Input: part model. Units: mm. Frame: model coordinates. A direction names the side the tool comes from. Give positions to 0.01 mm unless a question says otherwise; leave off trailing zeros. Loops run counter-clockwise (first coordinate to the right, second up) from the corner with the lowest first, then second, coordinate; pieces in that order, holes last. Notation, with made-up numbers: M 86.25,87.25 L 93.25,87.25 A27 cw 93.25,116.25 Z; hole C 13.5,58.5 d10. An arc over 180 degrees is marked long. Answer as a JSON object with one key per item and string values. Group by question number.
```python
from build123d import *
from build123d.topology import SkipClean

# Parameters (mm, degrees)
SKETCH1_R               = 16.65
BOSS_EXTRUDE1_DEPTH     = 2.5
SKETCH2_R               = 15.15
BOSS_EXTRUDE2_DEPTH     = 1.3
SKETCH3_R               = 16.65
BOSS_EXTRUDE3_DEPTH     = 27
CUT_EXTRUDE1_DEPTH      = 27
CUT_EXTRUDE1_DEPTH_BACK = 27
CUT_EXTRUDE2_DEPTH      = 26
CUT_EXTRUDE3_DEPTH      = 12.5
BOSS_EXTRUDE4_START     = -7
SKETCH8_R               = 4
BOSS_EXTRUDE4_DEPTH     = 10.5
FILLET1_R               = 3
SKETCH9_R               = 4
CUT_EXTRUDE4_DEPTH      = 33.5
CUT_EXTRUDE5_DEPTH      = 2
SKETCH11_R              = 15.35
CUT_EXTRUDE6_DEPTH      = 4


with BuildPart() as part:
    # Sketch1 → Boss-Extrude1 (new body)
    with BuildSketch(Plane(origin=(0, 0, 0), x_dir=(1, 0, 0), z_dir=(0, 1, 0))):
        with Locations(Location((0, 0, 0), (0, 0, 270))):
            Circle(SKETCH1_R)
    extrude(amount=BOSS_EXTRUDE1_DEPTH)

    # Sketch2 → Boss-Extrude2 (add)
    with BuildSketch(Plane(origin=(0, 2.5, 0), x_dir=(1, 0, 0), z_dir=(0, 1, 0))):
        with Locations(Location((0, 0, 0), (0, 0, 270))):
            Circle(SKETCH2_R)
    extrude(amount=BOSS_EXTRUDE2_DEPTH)

    # Sketch3 → Boss-Extrude3 (add)
    with BuildSketch(Plane(origin=(0, 3.8, 0), x_dir=(1, 0, 0), z_dir=(0, 1, 0))):
        with Locations(Location((0, 0, 0), (0, 0, 270))):
            Circle(SKETCH3_R)
    extrude(amount=BOSS_EXTRUDE3_DEPTH)

    # Sketch4 → Cut-Extrude1 (cut, two sides: drawn at the far end of the back side and taken through both)
    with BuildSketch(Plane.XY.offset(-CUT_EXTRUDE1_DEPTH_BACK)):
        with BuildLine():
            Line((-12.15, 30.8), (-10.299201712, 28.949201712))
            ThreePointArc((-10.299201712, 28.949201712), (-9.001508317, 28.082110707), (-7.470774587, 27.777628837))
            Line((-7.470774587, 27.777628837), (7.470774587, 27.777628837))
            ThreePointArc((7.470774587, 27.777628837), (9.001508317, 28.082110707), (10.299201712, 28.949201712))
            Line((10.299201712, 28.949201712), (12.15, 30.8))
            Line((12.15, 30.8), (-12.15, 30.8))
        make_face()
    extrude(amount=CUT_EXTRUDE1_DEPTH + CUT_EXTRUDE1_DEPTH_BACK, mode=Mode.SUBTRACT)

    # Sketch6 → Cut-Extrude2 (cut)
    with BuildSketch(Plane(origin=(0, 30.8, 0), x_dir=(1, 0, 0), z_dir=(0, 1, 0))):
        with BuildLine():
            Line((-12.249897959, 9.25), (12.249897959, 9.25))
            ThreePointArc((12.249897959, 9.25), (15.35, 0), (12.249897959, -9.25))
            Line((12.249897959, -9.25), (-12.249897959, -9.25))
            ThreePointArc((-12.249897959, -9.25), (-15.35, 0), (-12.249897959, 9.25))
        make_face()
    extrude(amount=-CUT_EXTRUDE2_DEPTH, mode=Mode.SUBTRACT)

    # Sketch7 → Cut-Extrude3 (cut)
    with BuildSketch(Plane.XY.offset(24.5)):
        with BuildLine():
            Line((-9.3, 6.2), (9.3, 6.2))
            ThreePointArc((9.3, 6.2), (10.714213562, 6.785786438), (11.3, 8.2))
            Line((11.3, 8.2), (11.3, 19.5))
            ThreePointArc((11.3, 19.5), (10.714213562, 20.914213562), (9.3, 21.5))
            Line((9.3, 21.5), (-9.3, 21.5))
            ThreePointArc((-9.3, 21.5), (-10.714213562, 20.914213562), (-11.3, 19.5))
            Line((-11.3, 19.5), (-11.3, 8.2))
            ThreePointArc((-11.3, 8.2), (-10.714213562, 6.785786438), (-9.3, 6.2))
        make_face()
    cut_extrude3 = extrude(amount=-CUT_EXTRUDE3_DEPTH, mode=Mode.SUBTRACT)

    # Mirror1: Cut-Extrude3 across plane
    add(cut_extrude3.mirror(Plane.XY), mode=Mode.SUBTRACT)

    # Sketch8 → Boss-Extrude4 (add)
    with BuildSketch(Plane(origin=(0, 0, -12), x_dir=(-1, 0, 0), z_dir=(0, 0, -1)).offset(BOSS_EXTRUDE4_START)):
        with BuildLine():
            Line((-2.837252192, 21.5), (2.837252192, 21.5))
            ThreePointArc((2.837252192, 21.5), (0, 10), (-2.837252192, 21.5))
        make_face()
        with Locations((0, 16.1)):
            Circle(SKETCH8_R, mode=Mode.SUBTRACT)
    boss_extrude4 = extrude(amount=BOSS_EXTRUDE4_DEPTH)

    # Mirror2: Boss-Extrude4 across plane
    add(boss_extrude4.mirror(Plane.XY))

    # Fillet1
    fillet1_edges = [part.edges().sort_by_distance(p)[0] for p in [
        (15.35, 4.8, 0),
        (0, 4.8, 9.25),
        (-15.35, 4.8, 0),
        (0, 4.8, -9.25),
    ]]
    fillet(fillet1_edges, radius=FILLET1_R)

    # Sketch9 → Cut-Extrude4 (cut)
    with BuildSketch(Plane(origin=(0, 0, -12), x_dir=(-1, 0, 0), z_dir=(0, 0, -1))):
        with Locations((0, 16.1)):
            Circle(SKETCH9_R)
    extrude(amount=-CUT_EXTRUDE4_DEPTH, mode=Mode.SUBTRACT)

    # Sketch10 → Cut-Extrude5 (cut)
    with SkipClean():  # the faces are left unmerged after this step: merging them gives an invalid solid
        with BuildSketch(Plane(origin=(0, 0, -12), x_dir=(-1, 0, 0), z_dir=(0, 0, -1))):
            with BuildLine():
                Line((0.611782833, 6.2), (0.611782833, 10.03075608))
                ThreePointArc((0.611782833, 10.03075608), (3.335542493, 10.992734952), (5.311313245, 13.100008065))
                Line((5.311313245, 13.100008065), (5.311313245, 6.2))
                Line((5.311313245, 6.2), (0.611782833, 6.2))
            make_face()
            with BuildLine():
                Line((-5.311313245, 6.2), (-5.311313245, 13.100008065))
                ThreePointArc((-5.311313245, 13.100008065), (-3.335542493, 10.992734952), (-0.611782833, 10.03075608))
                Line((-0.611782833, 10.03075608), (-0.611782833, 6.2))
                Line((-0.611782833, 6.2), (-5.311313245, 6.2))
            make_face()
        cut_extrude5 = extrude(amount=-CUT_EXTRUDE5_DEPTH, mode=Mode.SUBTRACT)

    # Mirror3: Cut-Extrude5 across plane
    with SkipClean():  # the faces are left unmerged after this step: merging them gives an invalid solid
        add(cut_extrude5.mirror(Plane.XY), mode=Mode.SUBTRACT)

    # Sketch11 → Cut-Extrude6 (cut)
    with BuildSketch(Plane(origin=(0, 30.8, 0), x_dir=(1, 0, 0), z_dir=(0, 1, 0))):
        with Locations(Location((0, 0, 0), (0, 0, 240.876388921))):
            Circle(SKETCH11_R)
    extrude(amount=-CUT_EXTRUDE6_DEPTH, mode=Mode.SUBTRACT)


solid = part.part
```
1. Mould query, pull axis Y, two halves, no side actions, for faces 1 (the flat face through (-8, 14, 12)), 2 (the flat face through (11.21, 29.86, -11.26)). Classes: pulls with the +Y half, pulls with the -Y half, needs draft (parallel to the pull), parting line crosses it, or undercut.
2. Section C-C (x = 0). Count the separate pieces of the cut face and the enclosed holes in it, then the cut area to 3 significant figures.
3. Section B-B (z = 0). Output: boundary loops of the cut face in (x, y), then the cut area to 3 significant figures.
4. Reachability of faces 3 (the flat face through (0, 6.2, 13)), 4 (the flat face through (0, 21.5, 7)), 5 (the flat face through (3, 9, -10)) from +Z, -Z, +X, -X, +Y, -Y: full face, straight path, thin tool, end or side. Return the list, or none.
5. First-contact query: P1, Ø5, axis at x = -3, y = 11.5, coming from the +Z side; P2, Ø6.5, axis at x = -3, z = -13, coming from the +Y side; P3, Ø1.6, axis at y = 8, z = -11.5, coming from the -X side. Flat tips, straight axial feed; report the tip coordinate or a pass-through.
6. Section A-A (y = 26). Output: boundary loops of the cut face in (x, z).
7. Material intervals for L1, parallel to Y at x = 0, z = -12.75; L2, parallel to X at y = 15.5, z = -8.5; L3, parallel to X at y = 16, z = -9, sorted ascending.
Geometry results:
{
 "1": {"face 1": "undercut", "face 2": "pulls with the +Y half"},
 "2": {"separate pieces": "3", "enclosed holes": "0", "area": "356 mm2"},
 "3": {"outline": "M -16.65,0 L 16.65,0 L 16.65,2.5 L 15.15,2.5 L 15.15,3.8 L 16.65,3.8 L 16.65,30.8 L 15.35,30.8 L 15.35,7.8 A3 cw 12.35,4.8 L -12.35,4.8 A3 cw -15.35,7.8 L -15.35,30.8 L -16.65,30.8 L -16.65,3.8 L -15.15,3.8 L -15.15,2.5 L -16.65,2.5 Z", "area": "227 mm2"},
 "4": {"face 3": "+Z", "face 4": "+Y", "face 5": "-Z"},
 "5": {"P1": "z = 15.5", "P2": "y = 27.78", "P3": "x = -12.76"},
 "6": {"outline": "C 0,0 d33.3; hole M -12.25,-9.25 L 12.25,-9.25 A15.35 ccw 12.25,9.25 L -12.25,9.25 A15.35 ccw Z"},
 "7": {"L1": "0 to 6.2, 10 to 12.1, 20.1 to 26.8", "L2": "-14.32 to -12.78, -6.07 to -3.95, 3.95 to 6.07, 12.78 to 14.32", "L3": "-14.01 to -12.43, -6.1 to -4, 4 to 6.1, 12.43 to 14.01"}
}
